Geometry check sheet. Reference: the model listing, model coordinates, mm. A direction names the side the tool comes from. Coordinates: 2 decimals unless noted, no trailing zeros. Write each loop counter-clockwise with the first axis right and the second up, starting at its lowest first coordinate (ties: lowest second). Pieces come first, ordered by that corner, then holes. Notation, with made-up numbers: (65, 8.25) -> (123, 8.25) arc R17 ccw to (123, 24.25) -> close; hole circle Ø2 at (-38.5, 84). An arc over 180 degrees is marked (long way). Answer in a Markdown table with one row per item. Add a question column.
1. Cross-section at D-D on x = 4. Record the cut outline in (y, z), and give its area (3 significant figures).
2. Mould release check, pull along X, two halves, no side actions. Record for faces 1 (the cylindrical face through (12.931, -8.035, 5.355)), 2 (the cylindrical face through (12.62, -8.89, 5.49)), 3 (the flat face through (-2.4, 6.245, 5.5)): pulls with the +X half, pulls with the -X half, needs draft (parallel to the pull), parting line crosses it, or undercut.
3. Depth check by flat-ended pin: P1, Ø0.5, axis at x = 17.5, z = 5.5, coming from the +Y side. Enter the tip coordinate at first touch or a pass-through.
4. Cross-section at C-C on y = -3.5. Record the cut outline in (x, z), and give its area (3 significant figures).
5. Set-up check for faces 4 (the flat face through (16.4, 4.013, 5.5)), 5 (the flat face through (-2.4, -6.286, 5.5)), 6 (the conical face through (12.962, -8.145, 5.815)), 7 (the cylindrical face through (12.8, 6.95, 5.35)): record each of +Z, -Z, +X, -X, +Y, -Y from which the full face is reachable in a straight line by a thin tool's end or side.
6. Cross-section at A-A on z = 5.3. Record the cut outline in (x, y), and give its area (3 significant figures).
7. Scan lines: L1, parallel to Y at x = 12, z = 5.8; L2, parallel to Y at x = 12.75, z = 5.15; L3, parallel to Y at x = 16, z = 5.6. Record each from-to range of solid material in increasing order. Write a range as from..to.
8. Cross-section at B-B on x = 10.5. Give the number of separate pieces and of enclosed holes in the cut face, and give its area (3 significant figures).
```python
from build123d import *

# Parameters (mm, degrees)
PAD002_DEPTH    = 1
SKETCH007_R     = 1.692877
POCKET001_DEPTH = 1
SKETCH008_R     = 1.73446
POCKET002_DEPTH = 1
CHAMFER_SIZE    = 0.5
POCKET005_DEPTH = 5
SKETCH009_W     = 8.212181
SKETCH009_H     = 8.085074
POCKET006_DEPTH = 5
FILLET004_R     = 0.3
FILLET005_R     = 0.3
CHAMFER001_SIZE = 0.3
CHAMFER002_SIZE = 0.3


with BuildPart() as part:
    # Sketch006 → Pad002 (new body)
    with BuildSketch(Plane.XY.offset(5)):
        with BuildLine():
            Line((-9.568426, -6.285917), (4.972526, -6.285917))
            ThreePointArc((4.972526, -6.285917), (20.334041, -0.01843), (4.970857, 6.244966))
            Line((-9.568426, 6.244966), (4.970857, 6.244966))
            Line((-9.568426, -6.285917), (-9.568426, 6.244966))
        make_face()
    extrude(amount=PAD002_DEPTH)

    # Sketch007 (on Pad) → Pocket001 (cut)
    with BuildSketch(Plane.XY.offset(5)):
        with Locations((-2.957902, 0.204839)):
            Circle(SKETCH007_R)
    extrude(amount=-POCKET001_DEPTH, mode=Mode.SUBTRACT)

    # Sketch008 (on Face6 of Pad002) → Pocket002 (cut)
    with BuildSketch(Plane.XY.offset(6)):
        with Locations((-2.984237, 0.234427)):
            Circle(SKETCH008_R)
    extrude(amount=-POCKET002_DEPTH, mode=Mode.SUBTRACT)

    # Chamfer
    chamfer_edges = [part.edges().sort_by_distance(p)[0] for p in [
        (-4.718697, 0.234427, 6),
    ]]
    chamfer(chamfer_edges, length=CHAMFER_SIZE)

    # Sketch011 → Pocket005 (cut)
    with BuildSketch(Plane.XY.offset(6)):
        with BuildLine():
            ThreePointArc((16.954988, 6.278391), (13.004004, 8.225263), (8.611476, 7.899254))
            Line((8.611476, 7.899254), (9.109037, 6.707427))
            ThreePointArc((16.036381, 5.369056), (12.751013, 6.961134), (9.109037, 6.707427))
            Line((16.954988, 6.278391), (16.036381, 5.369056))
        make_face()
        with BuildLine():
            ThreePointArc((8.677646, -7.709712), (12.991395, -8.023159), (16.861761, -6.092627))
            Line((15.900234, -5.234123), (16.861761, -6.092627))
            ThreePointArc((9.154517, -6.521003), (12.69888, -6.776571), (15.900234, -5.234123))
            Line((8.677646, -7.709712), (9.154517, -6.521003))
        make_face()
    extrude(amount=-POCKET005_DEPTH, mode=Mode.SUBTRACT)

    # Sketch009 (on Face1 of Chamfer) → Pocket006 (cut)
    with BuildSketch(Plane.XY.offset(6)):
        with Locations((17.565425, -0.029473)):
            Rectangle(SKETCH009_W, SKETCH009_H)
    extrude(amount=-POCKET006_DEPTH, mode=Mode.SUBTRACT)

    # Fillet004
    fillet004_edges = [part.edges().sort_by_distance(p)[0] for p in [
        (12.69888, -6.776571, 6),
    ]]
    fillet(fillet004_edges, radius=FILLET004_R)

    # Fillet005
    fillet005_edges = [part.edges().sort_by_distance(p)[0] for p in [
        (12.751013, 6.961134, 6),
    ]]
    fillet(fillet005_edges, radius=FILLET005_R)

    # Chamfer001
    chamfer001_edges = [part.edges().sort_by_distance(p)[0] for p in [
        (12.991395, -8.023159, 6),
    ]]
    chamfer(chamfer001_edges, length=CHAMFER001_SIZE)

    # Chamfer002
    chamfer002_edges = [part.edges().sort_by_distance(p)[0] for p in [
        (13.004004, 8.225263, 6),
    ]]
    chamfer(chamfer002_edges, length=CHAMFER002_SIZE)


solid = part.part
```
Results found:
| question | item | result |
|---|---|---|
| 1 | outline | (-6.29, 5) -> (6.24, 5) -> (6.24, 6) -> (-6.29, 6) -> close |
| 1 | area | 12.5 mm^2 |
| 2 | face 1 | undercut |
| 2 | face 2 | parting line crosses it |
| 2 | face 3 | needs draft |
| 3 | P1 | stops at y = 6.74 |
| 4 | outline | (-9.57, 5) -> (13.46, 5) -> (13.46, 6) -> (-9.57, 6) -> close |
| 4 | area | 23.0 mm^2 |
| 5 | face 4 | +Z, -Z, +X |
| 5 | face 5 | +Z, -Z, -X, -Y |
| 5 | face 6 | +Z |
| 5 | face 7 | +Z, -Z |
| 6 | outline | (-9.57, -6.29) -> (4.97, -6.29) arc R8.96 ccw to (19.37, -4.07) -> (13.46, -4.07) -> (13.46, 4.01) -> (19.38, 4.01) arc R8.96 ccw to (4.97, 6.24) -> (-9.57, 6.24) -> close; hole circle Ø3.47 at (-2.98, 0.23); hole (8.61, 7.9) -> (9.11, 6.71) arc R7.09 cw to (16.04, 5.37) -> (16.95, 6.28) arc R8.38 ccw to start; hole (8.68, -7.71) arc R8.18 ccw to (16.86, -6.09) -> (15.9, -5.23) arc R6.9 cw to (9.15, -6.52) -> close |
| 6 | area | 329 mm^2 |
| 7 | L1 | y = -8.96..-8.26, -6.86..7.05, 8.46..8.92 |
| 7 | L2 | y = -8.87..-8.07, -6.77..6.96, 8.27..8.83 |
| 7 | L3 | y = -7.69..-6.77, -5.32..-4.07, 4.01..5.4, 7.01..7.65 |
| 8 | separate pieces | 3 |
| 8 | enclosed holes | 0 |
| 8 | area | 15.1 mm^2 |
